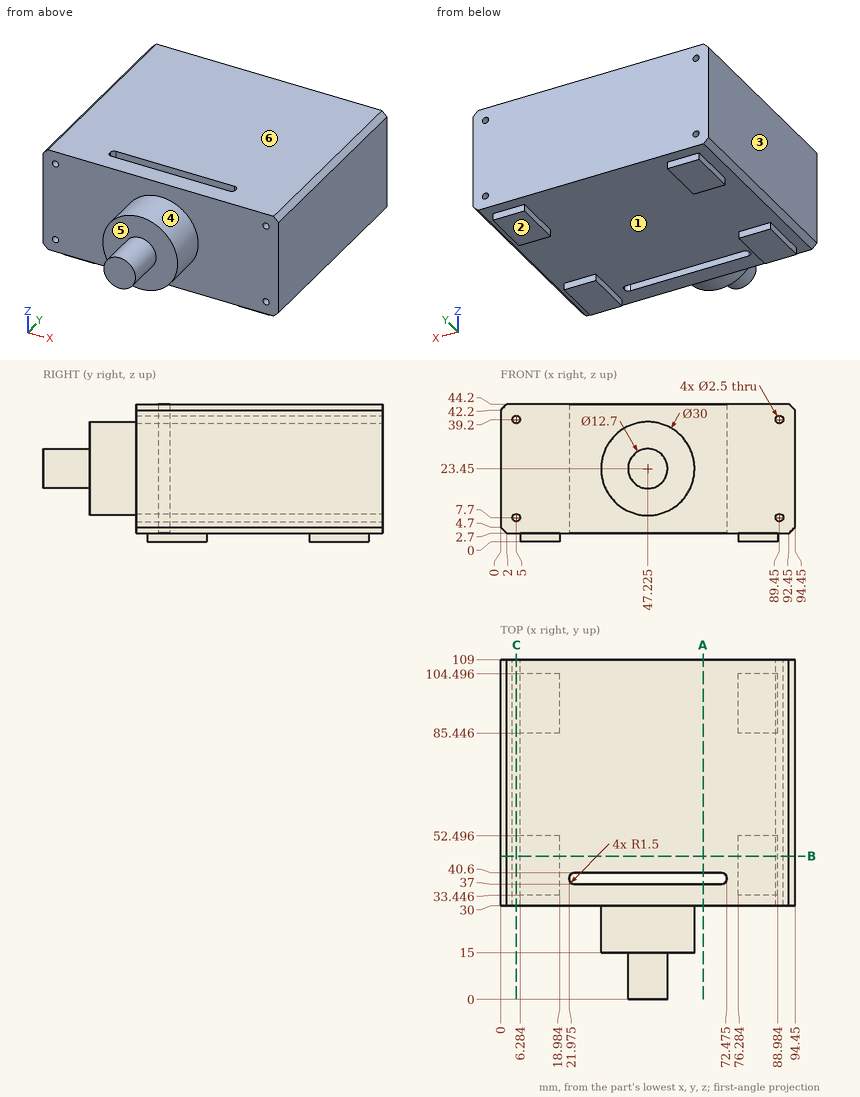
Part print with two shaded views. Sizes in mm from the minimum x, y, z corner. A direction names the side the tool comes from. Round coordinates to 2 decimals unless told otherwise and drop trailing zeros. Order: outer loops, then holes, each group sorted by start corner. A loop starts at its lowest first (then second) coordinate and runs counter-clockwise, first axis right, second up. Notation, with made-up numbers: M 81,-25 L 119,-25 A12 cw 119,-20 Z; hole C 81,81 d5. An arc over 180 degrees is marked long. Put each result on its own line as item: value. Start each with the question number.
1. Slice it at C-C on x = 5. List the corners of the cut face in (y, z), then the cut area to 3 significant figures.
2. Slice it at A-A on x = 65. List the corners of the cut face in (y, z).
3. Drill centre lines: probe 1 along Z at (x, y) = (5, 48.5); probe 2 along Y at (x, z) = (36.5, 38); probe 3 along Y at (x, z) = (49, 16). Where is each one in solid material? Low to high. Write a range as [from, to].
4. Two-plate mould, pull along X, no slides. Class the marked faces 1, 2, 3 and 4: +X half, -X half, draft (parallel to the pull), parting line (faces both ways), or undercut.
5. Slice it at B-B on y = 46. List the corners of the cut face in (x, z), then the cut area to 3 significant figures.
6. Tool access for the marked faces 5 and 6: list every direction of +Z, -Z, +X, -X, +Y, -Y with a clear straight run to the whole face (end or side of a thin tool).
7. Drop flat-ended pins along their axis: pin 1 (2 mm diameter, centred on y = 97, z = 1.5, fed in from -X); pin 2 (0.8 mm diameter, centred on x = 83, z = 2, fed in from -Y); pin 3 (8 mm diameter, centred on x = 58.5, z = 38.5, fed in from -Y); pin 4 (2 mm diameter, centred on x = 5, z = 39.2, fed in from +Y). Give the stop position or say it passes through.
Findings:
1. outline: M 30,2.7 L 109,2.7 L 109,6.45 L 30,6.45 Z; M 30,8.95 L 109,8.95 L 109,37.95 L 30,37.95 Z; M 30,40.45 L 109,40.45 L 109,44.2 L 30,44.2 Z
1. area: 2,880 mm2
2. outline: M 30,2.7 L 37,2.7 L 37,44.2 L 30,44.2 Z; M 40.6,2.7 L 109,2.7 L 109,44.2 L 40.6,44.2 Z
3. probe 1: [2.7, 6.45], [8.95, 37.95], [40.45, 44.2]
3. probe 2: [30, 37], [40.6, 109]
3. probe 3: [15, 37], [40.6, 109]
4. face 1: undercut
4. face 2: draft
4. face 3: -X half
4. face 4: parting line
5. outline: M 0,4.7 L 2,2.7 L 6.28,2.7 L 6.28,0 L 18.98,0 L 18.98,2.7 L 76.28,2.7 L 76.28,0 L 88.98,0 L 88.98,2.7 L 92.45,2.7 L 94.45,4.7 L 94.45,42.2 L 92.45,44.2 L 2,44.2 L 0,42.2 Z; hole C 5,7.7 d2.5; hole C 5,39.2 d2.5; hole C 89.45,7.7 d2.5; hole C 89.45,39.2 d2.5
5. area: 3,960 mm2
6. face 5: -Y
6. face 6: +Z, +X, -X, +Y, -Y
7. pin 1: x = 6.28
7. pin 2: y = 33.45
7. pin 3: y = 15
7. pin 4: through
